Could you check a few things on this model? Use its own coordinates, in mm. Face numbers are marked on the shaded views. A direction names the side the tool comes from. Coordinates: 2 decimals unless noted, no trailing zeros. Write each loop counter-clockwise with the first axis right and the second up, starting at its lowest first coordinate (ties: lowest second). Pieces come first, ordered by that corner, then holes. Notation, with made-up numbers: (61, -3) - (115, -3) arc R26 cw to (115, 35) - close; hole circle Ø8 at (-18, -16). An arc over 180 degrees is marked (long way). Answer as a JSON object with one key per item and string values. Group by question number.
1) If we section it at B-B (x = 3): Write out the boundary of the cut face in (y, z).
2) If we section it at C-C (y = 25): Write out the boundary of the cut face in (x, z).
3) If we section it at D-D (x = 14.5): Write out the boundary of the cut face in (y, z).
4) We'd pull the mould along Z, two halves only. Please class the marked faces 5, 6 and 7: released by +Z, released by -Z, zero draft, split by the parting line, or undercut.
5) Please list where these lines run through material, in increasing order: line 1 along X through (y, z) = (0.9, -10); line 2 along Z through (x, y) = (-3, 2.2); line 3 along X through (y, z) = (28.5, -44).
6) Will these pins go through, and if not, where does the flat tip stop? pin 1 Ø4 at (x, y) = (19.5, 13.5) entering from +Z; pin 2 Ø1.8 at (x, z) = (-2, -11.5) entering from +Y; pin 3 Ø0.8 at (x, y) = (-3, 2) entering from -Z; pin 4 Ø18 at (x, z) = (24, -35.5) entering from -Y.
7) On a 3-axis mill with a long thin cutter (end or side, diameter ignored), from which of +Z, -Z, +X, -X, +Y, -Y can I reach the whole of each face in a straight line? I mean the marked faces 1, 2, 3 and 4. Say none if no direction works.
8) If we section it at A-A (z = -10): Write out the boundary of the cut face in (x, y), plus the area to 3 significant figures.
```python
from build123d import *

# Parameters (mm, degrees)
SKETCH1_W               = 40
SKETCH1_H               = 50
BOSS_EXTRUDE1_DEPTH     = 15
SKETCH2_W               = 16
SKETCH2_H               = 3
CUT_EXTRUDE1_DEPTH      = 10
SKETCH3_W               = 36
SKETCH3_H               = 45
CUT_EXTRUDE2_DEPTH      = 12.5
SKETCH4_W               = 40
SKETCH4_H               = 2.515653855
BOSS_EXTRUDE2_DEPTH     = 27.5
CUT_EXTRUDE3_DEPTH      = 70.686799324
SKETCH6_W               = 2
SKETCH6_H               = 17.5
SKETCH6_H_2             = 20
BOSS_EXTRUDE3_DEPTH     = 27.5
CUT_EXTRUDE5_DEPTH      = 77.852130745
CUT_EXTRUDE5_DEPTH_BACK = 77.852130745
SKETCH8_W               = 15
SKETCH8_H               = 3
BOSS_EXTRUDE4_DEPTH     = 6
SKETCH9_R               = 1.6
CUT_EXTRUDE6_DEPTH      = 79.589121385
FILLET1_R               = 2.5
CHAMFER3_SIZE           = 15


with BuildPart() as part:
    # Sketch1 → Boss-Extrude1 (new body)
    with BuildSketch(Plane(origin=(0, 0, 0), x_dir=(1, 0, 0), z_dir=(0, 1, 0))):
        with Locations((20, 25)):
            Rectangle(SKETCH1_W, SKETCH1_H)
    extrude(amount=BOSS_EXTRUDE1_DEPTH)

    # Sketch2 → Cut-Extrude1 (cut)
    with BuildSketch(Plane.XZ):
        with Locations((20, -1.5)):
            Rectangle(SKETCH2_W, SKETCH2_H)
    extrude(amount=-CUT_EXTRUDE1_DEPTH, mode=Mode.SUBTRACT)

    # Sketch3 → Cut-Extrude2 (cut)
    with BuildSketch(Plane.XZ):
        with Locations((20, -25.5)):
            Rectangle(SKETCH3_W, SKETCH3_H)
    extrude(amount=-CUT_EXTRUDE2_DEPTH, mode=Mode.SUBTRACT)

    # Sketch4 → Boss-Extrude2 (add)
    with BuildSketch(Plane(origin=(0, 15, 0), x_dir=(1, 0, 0), z_dir=(0, 1, 0))):
        with Locations((20, 48.742173073)):
            Rectangle(SKETCH4_W, SKETCH4_H)
    extrude(amount=BOSS_EXTRUDE2_DEPTH)

    # Sketch5 → Cut-Extrude3 (cut, through all)
    with BuildSketch(Plane(origin=(0, 15, 0), x_dir=(1, 0, 0), z_dir=(0, 1, 0))):
        with BuildLine():
            Line((13.75, 47.484346145), (6.25, 47.484346145))
            ThreePointArc((6.25, 47.484346145), (4.25, 45.484346145), (6.25, 43.484346145))
            Line((6.25, 43.484346145), (13.75, 43.484346145))
            ThreePointArc((13.75, 43.484346145), (15.75, 45.484346145), (13.75, 47.484346145))
        make_face()
        with BuildLine():
            Line((33.25, 47.484346145), (25.75, 47.484346145))
            ThreePointArc((25.75, 47.484346145), (23.75, 45.484346145), (25.75, 43.484346145))
            Line((25.75, 43.484346145), (33.25, 43.484346145))
            ThreePointArc((33.25, 43.484346145), (35.25, 45.484346145), (33.25, 47.484346145))
        make_face()
    extrude(amount=-CUT_EXTRUDE3_DEPTH, mode=Mode.SUBTRACT)

    # Sketch6 → Boss-Extrude3 (add)
    with BuildSketch(Plane(origin=(0, 15, 0), x_dir=(1, 0, 0), z_dir=(0, 1, 0))):
        with Locations((1, 38.734346145)):
            Rectangle(SKETCH6_W, SKETCH6_H)
        with Locations((39, 37.484346145)):
            Rectangle(SKETCH6_W, SKETCH6_H_2)
    extrude(amount=BOSS_EXTRUDE3_DEPTH)

    # Sketch7 → Cut-Extrude5 (cut, two sides: drawn at the far end of the back side and taken through both)
    with BuildSketch(Plane.ZY.offset(-CUT_EXTRUDE5_DEPTH_BACK)):
        with BuildLine():
            Line((-48, 4), (-48, 0))
            Line((-48, 0), (-43, 0))
            Line((-43, 0), (-43, 4))
            ThreePointArc((-43, 4), (-45.5, 6.5), (-48, 4))
        make_face()
    extrude(amount=CUT_EXTRUDE5_DEPTH + CUT_EXTRUDE5_DEPTH_BACK, mode=Mode.SUBTRACT)

    # Sketch8 → Boss-Extrude4 (add)
    with BuildSketch(Plane(origin=(40, 0, 0), x_dir=(0, 0, -1), z_dir=(1, 0, 0))):
        with Locations((7.5, 1.5)):
            Rectangle(SKETCH8_W, SKETCH8_H)
    boss_extrude4 = extrude(amount=BOSS_EXTRUDE4_DEPTH)

    # Sketch9 → Cut-Extrude6 (cut, through all)
    with BuildSketch(Plane(origin=(0, 3, 0), x_dir=(1, 0, 0), z_dir=(0, 1, 0))):
        with Locations(Location((43, 10, 0), (0, 0, 270))):
            Circle(SKETCH9_R)
    cut_extrude6 = extrude(amount=-CUT_EXTRUDE6_DEPTH, mode=Mode.SUBTRACT)

    # Mirror1: Boss-Extrude4, Cut-Extrude6 across plane
    add(boss_extrude4.mirror(Plane.ZY.offset(-20)))
    add(cut_extrude6.mirror(Plane.ZY.offset(-20)), mode=Mode.SUBTRACT)

    # Fillet1
    fillet1_edges = [part.edges().sort_by_distance(p)[0] for p in [
        (40, 1.5, -15),
        (46, 1.5, 0),
        (46, 1.5, -15),
        (-6, 1.5, 0),
        (-6, 1.5, -15),
        (0, 1.5, -15),
    ]]
    fillet(fillet1_edges, radius=FILLET1_R)

    # Chamfer3
    chamfer3_edges = [part.edges().sort_by_distance(p)[0] for p in [
        (39, 42.5, -27.484346145),
        (1, 42.5, -29.984346145),
    ]]
    chamfer(chamfer3_edges, length=CHAMFER3_SIZE)


solid = part.part
```
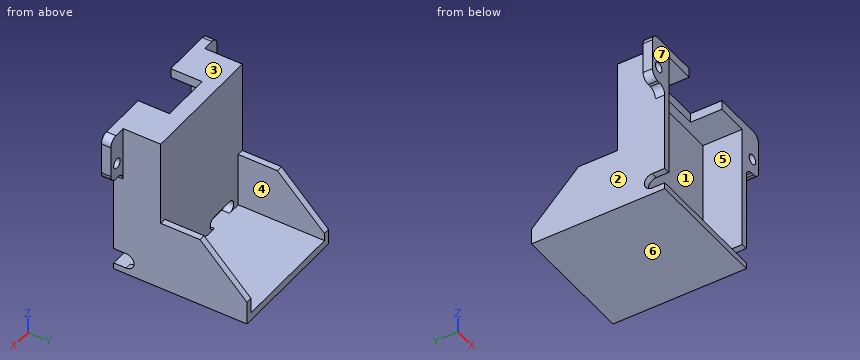
Here are the results:
{
 "1": {"outline": "(0, -50) - (42.5, -50) - (42.5, -47.48) - (15, -47.48) - (15, 0) - (0, 0) - (0, -3) - (12.5, -3) - (12.5, -48) - (0, -48) - close"},
 "2": {"outline": "(0, -50) - (40, -50) - (40, -27.48) - (38, -27.48) - (38, -47.48) - (2, -47.48) - (2, -29.98) - (0, -29.98) - close"},
 "3": {"outline": "(0, -50) - (42.5, -50) - (42.5, -47.48) - (15, -47.48) - (15, -47.34) - (12.5, -47.34) - (12.5, -48) - (0, -48) - close; (10, -3) - (12.5, -3) - (12.5, -43.63) - (15, -43.63) - (15, 0) - (10, 0) - close"},
 "4": {"face 5": "undercut", "face 6": "released by -Z", "face 7": "zero draft"},
 "5": {"line 1": "x = -6 to -4.6, -1.4 to 2, 38 to 41.4, 44.6 to 46", "line 2": "z = -15 to -11.6, -8.4 to 0", "line 3": "x = 0 to 2, 38 to 40"},
 "6": {"pin 1": "stops at z = 0", "pin 2": "stops at y = 3", "pin 3": "stops at z = -15", "pin 4": "stops at y = 12.5"},
 "7": {"face 1": "-Y", "face 2": "-Z, -X, +Y", "face 3": "+Z, +X, -X, +Y, -Y", "face 4": "+Z, +Y"},
 "8": {"outline": "(-6, 0) - (-4.6, 0) - (-4.6, 3) - (-6, 3) - close; (-1.4, 0) - (2, 0) - (2, 12.5) - (38, 12.5) - (38, 0) - (41.4, 0) - (41.4, 3) - (40, 3) - (40, 15) - (0, 15) - (0, 3) - (-1.4, 3) - close; (44.6, 0) - (46, 0) - (46, 3) - (44.6, 3) - close", "area": "167 mm²"}
}
